```python
from build123d import *

# Parameters (mm, degrees)
BOSS_EXTRUDE1_START = 0.762
SKETCH1_W           = 25.4
SKETCH1_H           = 19.05
BOSS_EXTRUDE1_DEPTH = 2.54
SKETCH2_W           = 24.638
SKETCH2_H           = 18.288
BOSS_EXTRUDE2_DEPTH = 0.762
BOSS_EXTRUDE3_DEPTH = 6.6675
BOSS_EXTRUDE4_DEPTH = 6.6675


with BuildPart() as part:
    # Sketch1 → Boss-Extrude1 (new body)
    with BuildSketch(Plane(origin=(0, 0, 0), x_dir=(1, 0, 0), z_dir=(0, 1, 0)).offset(BOSS_EXTRUDE1_START)):
        Rectangle(SKETCH1_W, SKETCH1_H)
    extrude(amount=BOSS_EXTRUDE1_DEPTH)

    # Sketch2 → Boss-Extrude2 (add)
    with BuildSketch(Plane.XZ.offset(-0.762)):
        Rectangle(SKETCH2_W, SKETCH2_H)
    extrude(amount=BOSS_EXTRUDE2_DEPTH)

    # Sketch4 → Boss-Extrude3 (add, symmetric)
    with BuildSketch(Plane.XY):
        with BuildLine():
            Line((1.501676205, 11.161675617), (3.533676205, 11.161675617))
            ThreePointArc((3.533676205, 11.161675617), (2.583870274, 7.696883923), (0, 5.200781521))
            Line((0, 5.200781521), (0, 3.302))
            Line((0, 3.302), (-4.28625, 3.302))
            Line((-4.28625, 3.302), (-4.28625, 4.445))
            ThreePointArc((-4.28625, 4.445), (-6.328557556, 5.099148106), (-8.06526082, 6.357238593))
            ThreePointArc((-8.06526082, 6.357238593), (-10.260478652, 13.572969866), (-5.489821493, 19.414766629))
            Line((-5.489821493, 19.414766629), (-5.561648074, 19.822115412))
            ThreePointArc((-5.561648074, 19.822115412), (-5.2081843, 22.205705846), (-4.060801058, 20.086755234))
            Line((-4.060801058, 20.086755234), (-4.022330337, 19.86857693))
            ThreePointArc((-4.022330337, 19.86857693), (-0.491642159, 19.803987548), (2.668342576, 18.227780941))
            Line((2.668342576, 18.227780941), (3.070034491, 18.719582328))
            Line((3.070034491, 18.719582328), (3.805281528, 17.090841988))
            Line((3.805281528, 17.090841988), (4.291759283, 17.499045293))
            Line((4.291759283, 17.499045293), (4.690845695, 15.752574138))
            Line((4.690845695, 15.752574138), (5.241166338, 16.07030191))
            Line((5.241166338, 16.07030191), (5.289319806, 14.273673387))
            Line((5.289319806, 14.273673387), (5.887168028, 14.491272344))
            Line((5.887168028, 14.491272344), (5.581577343, 12.720829512))
            Line((5.581577343, 12.720829512), (6.209142893, 12.831486251))
            Line((6.209142893, 12.831486251), (5.184676205, 10.780675617))
            Line((5.184676205, 10.780675617), (6.157416197, 10.780675617))
            Line((6.157416197, 10.780675617), (6.467196887, 7.825354003))
            ThreePointArc((6.467196887, 7.825354003), (5.725539877, 6.855170599), (4.714991862, 7.540811663))
            Line((4.714991862, 7.540811663), (3.439133103, 13.313172794))
            ThreePointArc((3.439133103, 13.313172794), (-5.274572471, 17.26630154), (-6.628419841, 7.794079572))
            ThreePointArc((-6.628419841, 7.794079572), (-1.438293949, 6.761699344), (1.501676205, 11.161675617))
        make_face()
    extrude(amount=BOSS_EXTRUDE3_DEPTH, both=True)

    # Sketch3 → Boss-Extrude4 (add, symmetric)
    with BuildSketch(Plane.XY):
        with BuildLine():
            Line((10.038311288, 3.302), (7.773782644, 11.753335954))
            Line((7.773782644, 11.753335954), (5.565676205, 11.161675617))
            Line((5.565676205, 11.161675617), (6.643306939, 13.028186801))
            Line((6.643306939, 13.028186801), (11.521611933, 14.335324685))
            ThreePointArc((11.521611933, 14.335324685), (13.628547334, 15.688756773), (13.232712451, 13.216051788))
            Line((13.232712451, 13.216051788), (9.245853603, 12.147776179))
            Line((9.245853603, 12.147776179), (11.616072187, 3.302))
            Line((11.616072187, 3.302), (10.038311288, 3.302))
        make_face()
    extrude(amount=BOSS_EXTRUDE4_DEPTH, both=True)


solid = part.part
```
The listing builds one solid part. Answer for the finished solid, in the listing's coordinates (mm). A direction names the side the tool comes from. Round coordinates to 2 decimals unless told otherwise and drop trailing zeros. Loops run counter-clockwise (first coordinate to the right, second up) from the corner with the lowest first, then second, coordinate; pieces in that order, holes last.
1) For faces 1 (the face through (4.49, 16.64, 0.09)), 2 (the face through (2, 11, 6.668)), 3 (the face through (6.31, 9.32, 0.09)), 4 (the face through (-10.28, 13.46, 0.09)), determine the directions among +Z, -Z, +X, -X, +Y, -Y from which every point of the face is accessible in a straight line to the end or side of a thin tool.
Outcome:
face 1: +Z, -Z, +Y
face 2: +Z, +X, -X, +Y
face 3: +Z, -Z
face 4: +Z, -Z, -X
2) Consider line 1 (X direction, y = 8, z = -3.5); line 2 (Y direction, x = 2.25, z = -5.25); line 3 (Y direction, x = -7.25, z = 4). Determine where each line is inside the solid, lowest interval first.
Outcome:
line 1: x = -9.33 to -6.82, 0.3 to 2.75, 4.61 to 6.45, 8.78 to 10.36
line 2: y = 0 to 3.3, 7.19 to 11.16, 15.78 to 18.55
line 3: y = 0 to 3.3, 5.66 to 8.52, 15.52 to 18.4
3) A cutting plane is placed at C-C on y = 16.75. Determine the outline of the cut face in (x, z).
Outcome:
outline: (-8.87, -6.67) - (-6.06, -6.67) - (-6.06, 6.67) - (-8.87, 6.67) - close; (1.26, -6.67) - (4.46, -6.67) - (4.46, 6.67) - (1.26, 6.67) - close
4) A cutting plane is placed at B-B on z = -7.75. Determine the outline of the cut face in (x, y), plus the area to 3 significant figures.
Outcome:
outline: (-12.7, 0.76) - (-12.32, 0.76) - (-12.32, 0) - (12.32, 0) - (12.32, 0.76) - (12.7, 0.76) - (12.7, 3.3) - (-12.7, 3.3) - close
area: 83.3 mm2
5) A cutting plane is placed at D-D on y = 9.25. Determine the outline of the cut face in (x, z), plus the area to 3 significant figures.
Outcome:
outline: (-9.92, -6.67) - (-7.7, -6.67) - (-7.7, 6.67) - (-9.92, 6.67) - close; (1.1, -6.67) - (3.26, -6.67) - (3.26, 6.67) - (1.1, 6.67) - close; (4.34, -6.67) - (6.32, -6.67) - (6.32, 6.67) - (4.34, 6.67) - close; (8.44, -6.67) - (10.02, -6.67) - (10.02, 6.67) - (8.44, 6.67) - close
area: 106 mm2
6) For a pull along X with two mould halves and no side action, classify faces 5 (the face through (0, 0, 0)), 6 (the face through (-5.252, 22.197, 0.093)), 7 (the face through (0, 4, 0)) as released by +X, released by -X, zero draft, split by the parting line, or undercut.
Outcome:
face 5: zero draft
face 6: split by the parting line
face 7: undercut
7) Given P1, Ø6, axis at x = 6, z = -7, coming from the -Y side; P2, Ø2.5, axis at x = 10, y = 8.5, coming from the -Z side; P3, Ø8, axis at x = -5.5, y = 12, coming from the +Z side; P4, Ø1, axis at y = 5.5, z = 7, coming from the -X side, each flat-ended and moving along its own axis, determine where each tip first touches the part or whether it passes through.
Outcome:
P1: stops at y = 0
P2: stops at z = -6.67
P3: stops at z = 6.67
P4: stops at x = -7.53
